Design review of the part built by this model. Coordinates are the model's own, in mm. A direction names the side the tool comes from. Coordinates: 2 decimals unless noted, no trailing zeros. Loops run counter-clockwise (first coordinate to the right, second up) from the corner with the lowest first, then second, coordinate; pieces in that order, holes last. Notation, with made-up numbers: (-3, 79.25) -> (42, 79.25) arc R36 ccw to (42, 116.25) -> close; hole circle Ø1 at (79.25, 45.25). An arc over 180 degrees is marked (long way). Use one line per item in the form item = value. Start each with the question number.
1. Consider section B-B (x = 450). State the section outline as (y, z) points, then the cut area to 3 significant figures.
2. The part is to be moulded in two halves that separate along Z. For faces 1 (the face through (8, 13, 11.43)), 2 (the face through (-8, 13, -12.7)), 3 (the face through (-8, 25.4, 0)), say which applies: released by +Z, released by -Z, zero draft, split by the parting line, or undercut.
3. Consider section A-A (z = 0.5). State the section outline as (x, y) points (3 decimals), then the cut area to 3 significant figures.
4. Machinability: for faces 4 (the face through (8, 24.13, 0)), 5 (the face through (-8, 13, 12.7)), which of the approach directions +Z, -Z, +X, -X, +Y, -Y give a long, thin tool a straight path to every point of the face, cutting with its end or side? Answer none if there is none.
5. Wall thickness on line 1 (Y direction, x = 297, z = -3.25); line 2 (Z direction, x = -149, y = 21.5): over which ranges is each line inside the solid? List them lowest first. Write a range as from..to.
6. Consider section C-C (y = 18.75). State the section outline as (x, z) points (3 decimals).
from build123d import *

# Parameters (mm, degrees)
BASE_W           = 1136.65
BASE_H           = 25.4
BOSS_FRAME_DEPTH = 25.4
SKETCH2_W        = 22.86
SKETCH2_H        = 22.86
CUT_HOLLOW_DEPTH = 1138.004693262
CUT_ANGLE_DEPTH  = 570.459064047


with BuildPart() as part:
    # Base → Boss-Frame (new body)
    with BuildSketch(Plane(origin=(0, 0, 0), x_dir=(1, 0, 0), z_dir=(0, 1, 0))):
        Rectangle(BASE_W, BASE_H)
    extrude(amount=BOSS_FRAME_DEPTH)

    # Sketch2 → Cut-Hollow (cut, through all)
    with BuildSketch(Plane(origin=(568.325, 0, 0), x_dir=(0, 0, -1), z_dir=(1, 0, 0))):
        with Locations((0, 12.7)):
            Rectangle(SKETCH2_W, SKETCH2_H)
    extrude(amount=-CUT_HOLLOW_DEPTH, mode=Mode.SUBTRACT)

    # Sketch4 → Cut-Angle (cut, through all)
    with BuildSketch(Plane.XY.offset(12.7)):
        Polygon((-568.325, 12.7), (-568.325, 0), (-555.645247213, 0), align=None)
        Polygon((568.325, 0), (555.645247213, 0), (568.325, 12.7), align=None)
    extrude(amount=-CUT_ANGLE_DEPTH, mode=Mode.SUBTRACT)


solid = part.part
Geometry check:
q1.outline = (0, -12.7) -> (25.4, -12.7) -> (25.4, 12.7) -> (0, 12.7) -> close; hole (1.27, -11.43) -> (24.13, -11.43) -> (24.13, 11.43) -> (1.27, 11.43) -> close
q1.area = 123 mm²
q2.face_1 = undercut
q2.face_2 = released by -Z
q2.face_3 = zero draft
q3.outline = (-568.325, 24.13) -> (568.325, 24.13) -> (568.325, 25.4) -> (-568.325, 25.4) -> close; (-556.913, 1.27) -> (-555.645, 0) -> (555.645, 0) -> (556.913, 1.27) -> close
q3.area = 2,860 mm²
q4.face_4 = +X, -X
q4.face_5 = +Z, +X, -X, +Y, -Y
q5.line_1 = 0..1.27, 24.13..25.4
q5.line_2 = -12.7..-11.43, 11.43..12.7
q6.outline = (-568.325, -12.7) -> (568.325, -12.7) -> (568.325, -11.43) -> (-568.325, -11.43) -> close; (-568.325, 11.43) -> (568.325, 11.43) -> (568.325, 12.7) -> (-568.325, 12.7) -> close
